The listing builds one solid part. Answer for the finished solid, in the listing's coordinates (mm). Face numbers are marked on the shaded views. A direction names the side the tool comes from. Round coordinates to 2 decimals unless told otherwise and drop trailing zeros. Order: outer loops, then holes, each group sorted by start corner. A loop starts at its lowest first (then second) coordinate and runs counter-clockwise, first axis right, second up. Notation, with made-up numbers: (48, 52.5) - (79, 52.5) arc R11 cw to (79, 68.5) - close; hole circle Ø3 at (-19, 46.5). An arc over 180 degrees is marked (long way). Write item = value, one per line.
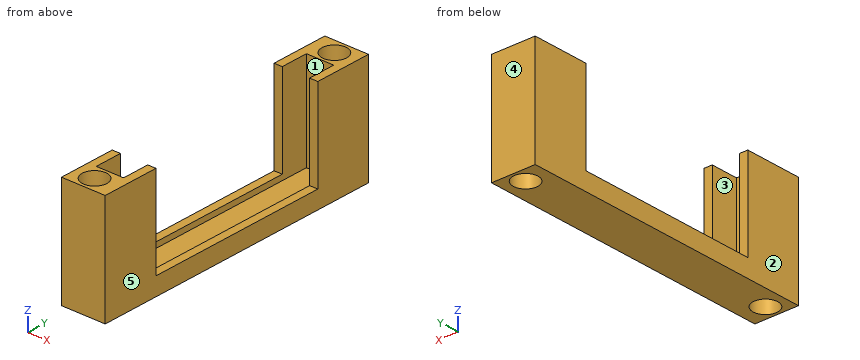
Autodesk Inventor part; units mm, degrees
ref_plane "YZ Plane" through (0, 0, 0) normal (1, 0, 0) x (0, 1, 0)
ref_plane "XZ Plane" through (0, 0, 0) normal (0, 1, 0) x (-1, 0, 0)
ref_plane "XY Plane" through (0, 0, 0) normal (0, 0, 1) x (1, 0, 0)
sketch "Sketch1" plane through (0, 0, 0) normal (0, 0, 1) x (1, 0, 0)
  line L0 (0, 0) -> (8, 0)
  line L1 (8, 0) -> (8, 50.5)
  line L2 (8, 50.5) -> (0, 50.5)
  line L3 (0, 50.5) -> (0, 0)
  dimension "d0" = 8
  dimension "d1" = 50.5
extrude "Extrusion1" add sketch "Sketch1" along normal blind 20
sketch "Sketch2" plane through (0, 0, 20) normal (0, 0, 1) x (1, 0, 0)
  line L0 (8, 0) -> (8, 50.5)
  line L1 (0, 42) -> (8, 42)
  line L2 (8, 42) -> (8, 8.5)
  line L3 (8, 8.5) -> (0, 8.5)
  line L4 (0, 8.5) -> (0, 42)
  line L5 (8, 50.5) -> (0, 50.5)
  line L6 (0, 0) -> (8, 0)
  dimension "d4" = 33.5
  dimension "d5" = 8.5
  dimension "d6" = 8.5
extrude "Extrusion2" cut sketch "Sketch2" against normal blind 16.74
sketch "Sketch3" plane through (0, 0, 20) normal (0, 0, 1) x (1, 0, 0)
  line L0 (1.5, 47) -> (6.5, 47)
  line L1 (6.5, 47) -> (6.5, 3.5)
  line L2 (6.5, 3.5) -> (1.5, 3.5)
  line L3 (1.5, 3.5) -> (1.5, 47)
  line L4 (0, 50.5) -> (0, 42)
  line L5 (0, 42) -> (8, 42)
  line L6 (8, 8.5) -> (0, 8.5)
  point P0 (0, 0)
  dimension "d9" = 5
  dimension "d10" = 1.5
  dimension "d11" = 5
  dimension "d12" = 5
extrude "Extrusion3" cut sketch "Sketch3" against normal blind 17.75
sketch "Sketch4" plane through (0, 0, 20) normal (0, 0, 1) x (1, 0, 0)
  line L0 (8, 50.5) -> (0, 50.5)
  line L1 (0, 50.5) -> (8, 50.5)
  line L2 (8, 50.5) -> (8, 52.5)
  line L3 (8, 52.5) -> (0, 52.5)
  line L4 (0, 52.5) -> (0, 50.5)
  line L5 (0, 0) -> (8, 0)
  line L6 (0, 0) -> (8, 0)
  line L7 (8, 0) -> (8, -2)
  line L8 (8, -2) -> (0, -2)
  line L9 (0, -2) -> (0, 0)
  dimension "d15" = 2
extrude "Extrusion4" add sketch "Sketch4" against normal up to surface (20 mm away)
sketch "Sketch5" plane through (0, 0, 20) normal (0, 0, 1) x (1, 0, 0)
  circle A0 centre (4.1899, 49.75) radius 2.25
  circle A1 centre (3.6194, 0.75) radius 2.25
  line L0 (0, -2) -> (8, -2)
  line L1 (6.5, 3.5) -> (1.5, 3.5)
  line L2 (1.5, 47) -> (6.5, 47)
  point P0 (0, 0)
  dimension "d18" = 5.5
  dimension "d19" = 4.5
  dimension "d20" = 2.75
  dimension "d21" = 2.75
extrude "Extrusion5" cut sketch "Sketch5" against normal up to surface (20 mm away)
properties part number "Stand Lower covet"
Q1. Section C-C on y = 28 is taken. Determine the outline of the cut face in (x, z), then the cut area to 3 significant figures.
Model answer:
outline = (0, 0) - (8, 0) - (8, 3.26) - (6.5, 3.26) - (6.5, 2.25) - (1.5, 2.25) - (1.5, 3.26) - (0, 3.26) - close
area = 21.0 mm^2
Q2. Determine the mould class of the marked faces 3, 4 and 5 for opening direction Y: released by +Y, released by -Y, zero draft, split by the parting line, or undercut.
Model answer:
face_3 = undercut
face_4 = released by +Y
face_5 = zero draft
Q3. Section D-D on x = 5.25 is taken. Determine the outline of the cut face in (y, z), then the cut area to 3 significant figures.
Model answer:
outline = (-2, 0) - (-0.8, 0) - (-0.8, 20) - (-2, 20) - close; (2.3, 0) - (47.77, 0) - (47.77, 20) - (47, 20) - (47, 2.25) - (3.5, 2.25) - (3.5, 20) - (2.3, 20) - close; (51.73, 0) - (52.5, 0) - (52.5, 20) - (51.73, 20) - close
area = 176 mm^2
Q4. For the marked faces 1 and 2, determine the directions among +Z, -Z, +X, -X, +Y, -Y from which every point of the face is accessible in a straight line to the end or side of a thin tool.
Model answer:
face_1 = +Z
face_2 = +Z, -Z, -X, +Y, -Y
Q5. A flat-ended cylindrical pin translates along its axis: P1, Ø1.2, axis at x = 7, y = 24, coming from the +Z side. Find the tip coordinate at first contact, or state that the pin passes through.
Model answer:
P1 = 3.26
Q6. Find the intervals of material crossed by line 1 (X direction, y = 5.5, z = 15.5); line 2 (Y direction, x = 4, z = 2); line 3 (Y direction, x = 3.75, z = 14), in increasing order. Write a range as from..to.
Model answer:
line_1 = 0..1.5, 6.5..8
line_2 = -2..-1.47, 2.97..47.51, 51.99..52.5
line_3 = -2..-1.5, 3..3.5, 47..47.54, 51.96..52.5
Q7. Section B-B on y = 0.75 is taken. Determine the outline of the cut face in (x, z).
Model answer:
outline = (0, 0) - (1.37, 0) - (1.37, 20) - (0, 20) - close; (5.87, 0) - (8, 0) - (8, 20) - (5.87, 20) - close
Q8. Section A-A on z = 17 is taken. Determine the outline of the cut face in (x, y).
Model answer:
outline = (0, -2) - (8, -2) - (8, 8.5) - (6.5, 8.5) - (6.5, 3.5) - (1.5, 3.5) - (1.5, 8.5) - (0, 8.5) - close; (0, 42) - (1.5, 42) - (1.5, 47) - (6.5, 47) - (6.5, 42) - (8, 42) - (8, 52.5) - (0, 52.5) - close; hole circle Ø4.5 at (3.62, 0.75); hole circle Ø4.5 at (4.19, 49.75)
